from build123d import *

# Parameters (mm, degrees)
F0_R          = 44.1944447312
F1_DEPTH      = 330.2
F2_T          = -15.24
F3_R          = 7.61999
F4_DEPTH      = 76.2
F5_SIZE       = 25.4
F6_W          = 80.8569788933
F6_H          = 113.4834885597
F7_DEPTH      = 63.5
F8_T1_DEPTH   = 240.4834885597
F8_T6_DEPTH   = 207.8569788933
F8_S7_R       = 44.1944447312
F8_T8_DEPTH   = 107
F8_T12_DEPTH  = 207.8569788933
F8_S13_R      = 44.1944447312
F8_T14_DEPTH  = 107
F10_DEPTH     = 10.16
F11_T4_DEPTH  = 181.6717263284
F11_S5_R      = 44.1944447312
F11_T6_DEPTH  = 95
F11_T10_DEPTH = 182.9126104381
F11_S11_R     = 44.1944447312
F11_T12_DEPTH = 95
F11_T16_DEPTH = 182.201088869
F11_S17_R     = 44.1944447312
F11_T18_DEPTH = 95
F11_T22_DEPTH = 180.9663017132
F11_S23_R     = 44.1944447312
F11_T24_DEPTH = 94


# Not quite as in the source:
# - a fillet or chamfer that OpenCascade refuses, or shapes differently, is made with other operations: its cross-section is extruded or revolved along the edge and cut away or added
# - a fillet or chamfer is up to 0.001 mm smaller than in the source, because OpenCascade refuses the exact size


with BuildPart() as f1:
    # F0 (on Front) → F1 (new body)
    with BuildSketch(Plane.XZ):
        Circle(F0_R)
    extrude(amount=F1_DEPTH)

    # F2
    f2_openings = [f1.faces().sort_by_distance(p)[0] for p in [
        (0, -330.2, 0),
    ]]
    offset(amount=F2_T, openings=f2_openings)

    # F3 (radius 7.62 in the source; OpenCascade refuses exactly that, so slightly less here)
    f3_edges = [f1.edges().sort_by_distance(p)[0] for p in [
        (-44.194445, -330.2, 0),
        (-28.954445, -330.2, 0),
    ]]
    fillet(f3_edges, radius=F3_R)

    # F4 (add): a face of the model
    f4_faces = [f1.faces().sort_by_distance(p)[0] for p in [
        (0, 0, 0),
    ]]
    extrude(f4_faces, amount=F4_DEPTH)

    # F5
    f5_edges = [f1.edges().sort_by_distance(p)[0] for p in [
        (-44.194445, 76.2, 0),
    ]]
    chamfer(f5_edges, length=F5_SIZE)

    # F6 (on Top) → F7 (join)
    with BuildSketch(Plane.XY):
        with Locations((0, -144.0225243568)):
            Rectangle(F6_W, F6_H)
    extrude(amount=F7_DEPTH)

    # F8: fillet of radius 25.4 on 4 edges, made by hand

    # F8_s2 → F8_t1 (cut)
    with BuildSketch(Plane.XZ.offset(23.780780077)):
        with BuildLine():
            ThreePointArc((40.4284894466, 38.1), (32.9890016888, 56.0605122421), (15.0284894466, 63.5))
            Line((15.0284894466, 63.5), (40.4284894466, 63.5))
            Line((40.4284894466, 63.5), (40.4284894466, 38.1))
        make_face()
        with BuildLine():
            ThreePointArc((-40.4284894466, 38.1), (-32.9890016888, 56.0605122421), (-15.0284894466, 63.5))
            Line((-15.0284894466, 63.5), (-40.4284894466, 63.5))
            Line((-40.4284894466, 63.5), (-40.4284894466, 38.1))
        make_face()
    extrude(amount=F8_T1_DEPTH, mode=Mode.SUBTRACT)


with BuildPart() as f8_tool4:
    # F8_s5 → F8_t6 (new body)
    with BuildSketch(Plane.YZ.offset(103.9284894466)):
        with BuildLine():
            ThreePointArc((-87.280780077, 38.1), (-94.7202678348, 56.0605122421), (-112.680780077, 63.5))
            Line((-112.680780077, 63.5), (-87.280780077, 63.5))
            Line((-87.280780077, 63.5), (-87.280780077, 38.1))
        make_face()
    extrude(amount=-F8_T6_DEPTH)

    # F8_s7 → F8_t8 (cut, symmetric)
    with BuildSketch(Plane.XZ.offset(100)):
        Circle(F8_S7_R)
    extrude(amount=F8_T8_DEPTH, both=True, mode=Mode.SUBTRACT)


with BuildPart() as f1_1:
    add(f1.part)

    # F8_t3: cut F8_tool4
    add(f8_tool4.part, mode=Mode.SUBTRACT)


with BuildPart() as f8_tool10:
    # F8_s11 → F8_t12 (new body)
    with BuildSketch(Plane.YZ.offset(-103.9284894466)):
        with BuildLine():
            ThreePointArc((-200.7642686367, 38.1), (-193.3247808788, 56.0605122421), (-175.3642686367, 63.5))
            Line((-175.3642686367, 63.5), (-200.7642686367, 63.5))
            Line((-200.7642686367, 63.5), (-200.7642686367, 38.1))
        make_face()
    extrude(amount=F8_T12_DEPTH)

    # F8_s13 → F8_t14 (cut, symmetric)
    with BuildSketch(Plane.XZ.offset(188.1)):
        Circle(F8_S13_R)
    extrude(amount=F8_T14_DEPTH, both=True, mode=Mode.SUBTRACT)


with BuildPart() as f1_2:
    add(f1_1.part)

    # F8_t9: cut F8_tool10
    add(f8_tool10.part, mode=Mode.SUBTRACT)

    # F9 (on Top) → F10 (join)
    with BuildSketch(Plane.XY):
        Polygon((181.1510026455, -156.4789265394), (181.1510026455, -86.3388031721), (-181.1510026455, -86.3388031721), (-181.1510026455, -156.4789265394), (-40.541768074, -156.4789265394), (40.4533445835, -156.4789265394), align=None)
        Polygon((40.4533445835, -200.733974576), (181.1510026455, -156.4789265394), (40.4533445835, -156.4789265394), align=None)
        Polygon((-40.541768074, -156.4789265394), (-181.1510026455, -156.4789265394), (-40.541768074, -198.22897017), align=None)
    extrude(amount=F10_DEPTH)

    # F11: fillet of radius 7.62 on 4 edges, made by hand


with BuildPart() as f11_tool2:
    # F11_s3 → F11_t4 (new body)
    with BuildSketch(Plane(origin=(-35.0743442089, -11.0322858902, 0), x_dir=(0, 0, 1), z_dir=(0.9539242957, 0.3000473932, 0))):
        with BuildLine():
            ThreePointArc((0, 196.0029358997), (2.2318463274, 201.3910895724), (7.62, 203.6229358997))
            Line((7.62, 203.6229358997), (0, 203.6229358997))
            Line((0, 203.6229358997), (0, 196.0029358997))
        make_face()
    extrude(amount=F11_T4_DEPTH)

    # F11_s5 → F11_t6 (cut, symmetric)
    with BuildSketch(Plane.XZ.offset(174.4)):
        Circle(F11_S5_R)
    extrude(amount=F11_T6_DEPTH, both=True, mode=Mode.SUBTRACT)


with BuildPart() as f1_3:
    add(f1_2.part)

    # F11_t1: cut F11_tool2
    add(f11_tool2.part, mode=Mode.SUBTRACT)


with BuildPart() as f11_tool8:
    # F11_s9 → F11_t10 (new body)
    with BuildSketch(Plane(origin=(-36.2580537092, -11.4046099325, 0), x_dir=(0, 0, 1), z_dir=(0.9539242957, 0.3000473932, 0))):
        with BuildLine():
            ThreePointArc((2.54, 203.6229358997), (7.9281536726, 201.3910895724), (10.16, 196.0029358997))
            Line((10.16, 196.0029358997), (10.16, 203.6229358997))
            Line((10.16, 203.6229358997), (2.54, 203.6229358997))
        make_face()
    extrude(amount=F11_T10_DEPTH)

    # F11_s11 → F11_t12 (cut, symmetric)
    with BuildSketch(Plane.XZ.offset(174.6)):
        Circle(F11_S11_R)
    extrude(amount=F11_T12_DEPTH, both=True, mode=Mode.SUBTRACT)


with BuildPart() as f1_4:
    add(f1_3.part)

    # F11_t7: cut F11_tool8
    add(f11_tool8.part, mode=Mode.SUBTRACT)


with BuildPart() as f11_tool14:
    # F11_s15 → F11_t16 (new body)
    with BuildSketch(Plane(origin=(-142.0383828725, 42.1743898985, 0), x_dir=(0, 0, 1), z_dir=(0.9586344454, -0.2846401237, 0))):
        with BuildLine():
            ThreePointArc((10.16, 193.9489327682), (7.9281536726, 199.3370864408), (2.54, 201.5689327682))
            Line((2.54, 201.5689327682), (10.16, 201.5689327682))
            Line((10.16, 201.5689327682), (10.16, 193.9489327682))
        make_face()
    extrude(amount=F11_T16_DEPTH)

    # F11_s17 → F11_t18 (cut, symmetric)
    with BuildSketch(Plane.XZ.offset(173.3)):
        Circle(F11_S17_R)
    extrude(amount=F11_T18_DEPTH, both=True, mode=Mode.SUBTRACT)


with BuildPart() as f1_5:
    add(f1_4.part)

    # F11_t13: cut F11_tool14
    add(f11_tool14.part, mode=Mode.SUBTRACT)


with BuildPart() as f11_tool20:
    # F11_s21 → F11_t22 (new body)
    with BuildSketch(Plane(origin=(-142.0383828725, 42.1743898985, 0), x_dir=(0, 0, 1), z_dir=(0.9586344454, -0.2846401237, 0))):
        with BuildLine():
            ThreePointArc((7.62, 201.5689327682), (2.2318463274, 199.3370864408), (0, 193.9489327682))
            Line((0, 193.9489327682), (0, 201.5689327682))
            Line((0, 201.5689327682), (7.62, 201.5689327682))
        make_face()
    extrude(amount=F11_T22_DEPTH)

    # F11_s23 → F11_t24 (cut, symmetric)
    with BuildSketch(Plane.XZ.offset(173.2)):
        Circle(F11_S23_R)
    extrude(amount=F11_T24_DEPTH, both=True, mode=Mode.SUBTRACT)


with BuildPart() as f1_6:
    add(f1_5.part)

    # F11_t19: cut F11_tool20
    add(f11_tool20.part, mode=Mode.SUBTRACT)


solid = f1_6.part
Model file for the job. Use its own axes, mm. A direction names the side the tool comes from. Give positions to 0.01 mm unless a question says otherwise; leave off trailing zeros. Loops run counter-clockwise (first coordinate to the right, second up) from the corner with the lowest first, then second, coordinate; pieces in that order, holes last. Notation, with made-up numbers: (65.25, 9.5) -> (73.25, 9.5) arc R12 ccw to (73.25, 31.5) -> close; hole circle Ø9 at (-17.75, 23). An arc over 180 degrees is marked (long way). Use a Markdown table: item, result. Add a question column.
(1) Slice it at A-A on y = -138.5. List the corners of the cut face in (x, z).
(2) Tool access for faces 1 (the flat face through (-36, -200.764, 32)), 2 (the flat face through (111, -127, 10.16)), 3 (the flat face through (-36, -87.281, 32)): list every direction of +Z, -Z, +X, -X, +Y, -Y with a clear straight run to the whole face (end or side of a thin tool).
(3) Wall check: line 1 along X through (y, z) = (-258, 0); line 2 along Z through (x, y) = (0, -177.5); line 3 along X through (y, z) = (-314, -3). Give the ranges that are in metal, low to high.
(4) Slice it at C-C on y = -2. List the corners of the cut face in (x, z), and give its area (3 significant figures).
(5) Mould opens along X. For faces 4 (the flat face through (112, -127, 0)), 5 (the cylindrical face through (-33.19, -143.23, 55.86)), 6 (the flat face through (0, -143, 0)) say: +X half, -X half, draft (parallel to the pull), parting line (faces both ways), or undercut.
(6) Drop flat-ended pins along their axis: pin 1 Ø10 at (y, z) = (-166, 26) entering from +X; pin 2 Ø11 at (x, z) = (112, 7) entering from +Y; pin 3 Ø1 at (x, z) = (19, 10.5) entering from -Y. Give the stop position or say it passes through.
Filled sheet:
| question | item | result |
|---|---|---|
| 1 | outline | (-181.15, 0) -> (-44.19, 0) arc R44.19 ccw to (44.19, 0) -> (181.15, 0) -> (181.15, 10.16) -> (43.01, 10.16) arc R44.19 ccw to (40.43, 17.85) -> (40.43, 38.1) arc R25.4 ccw to (15.03, 63.5) -> (-15.03, 63.5) arc R25.4 ccw to (-40.43, 38.1) -> (-40.43, 17.85) arc R44.19 ccw to (-43.01, 10.16) -> (-181.15, 10.16) -> close; hole (-28.95, 0) arc R28.95 ccw to (28.95, 0) -> close |
| 2 | face 1 | +Z, -X, -Y |
| 2 | face 2 | +Z, +X, +Y, -Y |
| 2 | face 3 | +Z, -X, +Y |
| 3 | line 1 | -44.19 to -28.95, 28.95 to 44.19 |
| 3 | line 2 | -44.19 to -28.95, 0 to 63.41 |
| 3 | line 3 | -44.09 to -28.8, 28.8 to 44.09 |
| 4 | outline | circle Ø88.39 at (0, 0) |
| 4 | area | 6,140 mm2 |
| 5 | face 4 | draft |
| 5 | face 5 | -X half |
| 5 | face 6 | undercut |
| 6 | pin 1 | x = 40.43 |
| 6 | pin 2 | y = -86.34 |
| 6 | pin 3 | y = -200.76 |
